Could you check a few things on this model? Use its own coordinates, in mm. A direction names the side the tool comes from. Coordinates: 2 decimals unless noted, no trailing zeros. Loops run counter-clockwise (first coordinate to the right, second up) from the corner with the lowest first, then second, coordinate; pieces in that order, holes last. Notation, with made-up numbers: M 66.5,52.5 L 93.5,52.5 A17 ccw 93.5,84.5 Z; hole C 18,15 d11. An arc over 180 degrees is marked long. Write each question's results on one line, items separated by ' | '.
```python
from build123d import *

# Parameters (mm, degrees)
F1_DEPTH = 3
F4_DEPTH = 5
F5_R     = 1


# Not quite as in the source:
# - a fillet or chamfer that OpenCascade refuses, or shapes differently, is made with other operations: its cross-section is extruded or revolved along the edge and cut away or added
# - a feature of the source that left no trace in its solid (it failed there, or was rolled back) is left out


with BuildPart() as f1:
    # F0 (on Top) → F1 (new body)
    with BuildSketch(Plane.XY):
        Polygon((-22, -13), (-22, 13), (-37, 13), (-42, 8), (-42, -8), (-37, -13), align=None)
        with BuildLine():
            Line((-15, -10.5), (-15, 10.5))
            ThreePointArc((-15, 10.5), (-16.767766953, 11.232233047), (-17.5, 13))
            Line((-17.5, 13), (-22, 13))
            Line((-22, 13), (-22, -13))
            Line((-22, -13), (-17.5, -13))
            ThreePointArc((-17.5, -13), (-16.767766953, -11.232233047), (-15, -10.5))
        make_face()
        Polygon((37, 13), (22, 13), (22, -13), (37, -13), (42, -8), (42, 8), align=None)
        with BuildLine():
            Line((15, 19), (15, 15.5))
            ThreePointArc((15, 15.5), (16.767766953, 14.767766953), (17.5, 13))
            Line((17.5, 13), (22, 13))
            Line((22, 13), (22, 19))
            Line((22, 19), (15, 19))
        make_face()
        with BuildLine():
            Line((22, -13), (17.5, -13))
            ThreePointArc((17.5, -13), (16.767766953, -14.767766953), (15, -15.5))
            Line((15, -15.5), (15, -19))
            Line((15, -19), (22, -19))
            Line((22, -19), (22, -13))
        make_face()
        with BuildLine():
            Line((12.5, 13), (-12.5, 13))
            ThreePointArc((-12.5, 13), (-13.232233047, 11.232233047), (-15, 10.5))
            Line((-15, 10.5), (-15, -10.5))
            ThreePointArc((-15, -10.5), (-13.232233047, -11.232233047), (-12.5, -13))
            Line((-12.5, -13), (12.5, -13))
            ThreePointArc((12.5, -13), (13.232233047, -11.232233047), (15, -10.5))
            Line((15, -10.5), (15, 10.5))
            ThreePointArc((15, 10.5), (13.232233047, 11.232233047), (12.5, 13))
        make_face()
        with BuildLine():
            ThreePointArc((-15, -15.5), (-16.767766953, -14.767766953), (-17.5, -13))
            Line((-17.5, -13), (-22, -13))
            Line((-22, -13), (-22, -19))
            Line((-22, -19), (-15, -19))
            Line((-15, -19), (-15, -15.5))
        make_face()
        Polygon((-15, 34), (-15, 19), (15, 19), (15, 34), (10, 39), (-10, 39), align=None)
        Polygon((15, -19), (-15, -19), (-15, -34), (-10, -39), (10, -39), (15, -34), align=None)
        Polygon((-22, -19), (-22, -13), (-37, -13), (-42, -18), (-42, -39), (-20, -39), (-15, -34), (-15, -19), align=None)
        Polygon((-22, 19), (-15, 19), (-15, 34), (-20, 39), (-42, 39), (-42, 18), (-37, 13), (-22, 13), align=None)
        Polygon((15, 34), (15, 19), (22, 19), (22, 13), (37, 13), (42, 18), (42, 39), (20, 39), align=None)
        Polygon((37, -13), (22, -13), (22, -19), (15, -19), (15, -34), (20, -39), (42, -39), (42, -18), align=None)
        with BuildLine():
            ThreePointArc((-17.5, 13), (-16.767766953, 14.767766953), (-15, 15.5))
            Line((-15, 15.5), (-15, 19))
            Line((-15, 19), (-22, 19))
            Line((-22, 19), (-22, 13))
            Line((-22, 13), (-17.5, 13))
        make_face()
        with BuildLine():
            Line((12.5, -13), (-12.5, -13))
            ThreePointArc((-12.5, -13), (-13.232233047, -14.767766953), (-15, -15.5))
            Line((-15, -15.5), (-15, -19))
            Line((-15, -19), (15, -19))
            Line((15, -19), (15, -15.5))
            ThreePointArc((15, -15.5), (13.232233047, -14.767766953), (12.5, -13))
        make_face()
        with BuildLine():
            ThreePointArc((-15, 15.5), (-13.232233047, 14.767766953), (-12.5, 13))
            Line((-12.5, 13), (12.5, 13))
            ThreePointArc((12.5, 13), (13.232233047, 14.767766953), (15, 15.5))
            Line((15, 15.5), (15, 19))
            Line((15, 19), (-15, 19))
            Line((-15, 19), (-15, 15.5))
        make_face()
        with BuildLine():
            ThreePointArc((17.5, 13), (16.767766953, 11.232233047), (15, 10.5))
            Line((15, 10.5), (15, -10.5))
            ThreePointArc((15, -10.5), (16.767766953, -11.232233047), (17.5, -13))
            Line((17.5, -13), (22, -13))
            Line((22, -13), (22, 13))
            Line((22, 13), (17.5, 13))
        make_face()
    extrude(amount=F1_DEPTH)

    # F2: chamfer of 2 on 4 edges, made by hand

    # F2_s1 → F2_t2 (revolve, cut)
    with BuildSketch(Plane.XZ.offset(13)):
        Polygon((-12.5, 1), (-10.5, 3), (-12.5, 3), align=None)
    revolve(axis=Axis((-15, -13, 3), (0, 0, -1)), mode=Mode.SUBTRACT)

    # F2_s3 → F2_t4 (revolve, cut)
    with BuildSketch(Plane.YZ.offset(-15)):
        Polygon((15.5, 1), (17.5, 3), (15.5, 3), align=None)
    revolve(axis=Axis((-15, 13, 3), (0, 0, -1)), mode=Mode.SUBTRACT)

    # F2_s5 → F2_t6 (revolve, cut)
    with BuildSketch(Plane.XZ.offset(-13)):
        Polygon((17.5, 1), (19.5, 3), (17.5, 3), align=None)
    revolve(axis=Axis((15, 13, 3), (0, 0, -1)), mode=Mode.SUBTRACT)

    # F2_s7 → F2_t8 (revolve, cut)
    with BuildSketch(Plane.YZ.offset(15)):
        Polygon((-10.5, 1), (-8.5, 3), (-10.5, 3), align=None)
    revolve(axis=Axis((15, -13, 3), (0, 0, -1)), mode=Mode.SUBTRACT)

    # F0 (on Top) → F4 (join)
    with BuildSketch(Plane.XY):
        Polygon((-22, 19), (-15, 19), (-15, 34), (-20, 39), (-42, 39), (-42, 18), (-37, 13), (-22, 13), align=None)
        Polygon((-22, -13), (-22, 13), (-37, 13), (-42, 8), (-42, -8), (-37, -13), align=None)
        Polygon((-22, -19), (-22, -13), (-37, -13), (-42, -18), (-42, -39), (-20, -39), (-15, -34), (-15, -19), align=None)
        Polygon((15, -19), (-15, -19), (-15, -34), (-10, -39), (10, -39), (15, -34), align=None)
        Polygon((37, -13), (22, -13), (22, -19), (15, -19), (15, -34), (20, -39), (42, -39), (42, -18), align=None)
        Polygon((37, 13), (22, 13), (22, -13), (37, -13), (42, -8), (42, 8), align=None)
        Polygon((15, 34), (15, 19), (22, 19), (22, 13), (37, 13), (42, 18), (42, 39), (20, 39), align=None)
        Polygon((-15, 34), (-15, 19), (15, 19), (15, 34), (10, 39), (-10, 39), align=None)
    extrude(amount=F4_DEPTH)

    # F5
    f5_edges = [f1.edges().sort_by_distance(p)[0] for p in [
        (-22, 19, 4),
        (-22, -19, 4),
        (22, 19, 4),
        (22, -19, 4),
    ]]
    fillet(f5_edges, radius=F5_R)


solid = f1.part
```
(1) Will this pin go through, and if not, where does the flat tip stop? P1, Ø2, axis at x = -15.5, y = -8.5, coming from the +Z side.
Reported:
P1: stops at z = 3
(2) Imagine slicing it at A-A, the plane z = 2.2. State how many separate pieces and enclosed holes the cut face has, and give its area (3 significant figures).
Reported:
separate pieces: 1 | enclosed holes: 4 | area: 6,180 mm2
(3) Please list where these lines run through material, in increasing order: probe 1 along X at (y, z) = (1.5, 4.1); probe 2 along X at (y, z) = (35, 3.95); probe 3 along X at (y, z) = (-14, 0.75). Write a range as from..to.
Reported:
probe 1: x = -42..-22, 22..42 | probe 2: x = -42..-16, -14..14, 16..42 | probe 3: x = -38..-17.29, -12.71..12.71, 17.29..38
(4) Imagine slicing it at B-B, the plane x = 0. List the corners of the cut face in (y, z) for me, and give its area (3 significant figures).
Reported:
outline: M -39,0 L 39,0 L 39,5 L 19,5 L 19,3 L -19,3 L -19,5 L -39,5 Z | area: 314 mm2
(5) If we mould it in two halves opening along Y, with no side actions, what happens to faces 5 (the flat face through (42, 0, 2)), 6 (the flat face through (-39, -15, 2)), 7 (the flat face through (-12, 37, 2)), 8 (the flat face through (39, -11, 2))? For each: released by +Y, released by -Y, zero draft, split by the parting line, or undercut.
Reported:
face 5: zero draft | face 6: undercut | face 7: released by +Y | face 8: undercut
(6) Which directions (+Z, -Z, +X, -X, +Y, -Y) give clear straight access to the entire face, cutting with the end or side of a thin tool? Please do faces 1 (the flat face through (-40, 16, 2)), 2 (the flat face through (0, 19, 4)), 3 (the flat face through (-18, -37, 2)), 4 (the flat face through (40, -16, 2)).
Reported:
face 1: +Z, -Z, -X | face 2: +Z | face 3: +Z, -Z, -Y | face 4: +Z, -Z, +X
